from build123d import *

# Parameters (mm, degrees)
SKETCH1_W           = 146.05
SKETCH1_H           = 101.6
BOSS_EXTRUDE1_DEPTH = 2.54
CUT_EXTRUDE1_DEPTH  = 178.931487095
SKETCH4_W           = 40.64
SKETCH4_H           = 95.25
SKETCH4_R           = 4.445
SKETCH4_R_2         = 4.7625
BOSS_EXTRUDE2_DEPTH = 2.54


with BuildPart() as part:
    # Sketch1 → Boss-Extrude1 (new body)
    with BuildSketch(Plane.XY):
        with Locations((73.025, -50.8)):
            Rectangle(SKETCH1_W, SKETCH1_H)
    extrude(amount=BOSS_EXTRUDE1_DEPTH)

    # Sketch2 → Cut-Extrude1 (cut, through all)
    with BuildSketch(Plane.XY):
        with BuildLine():
            Line((80.01, -72.39), (41.91, -72.39))
            Line((41.91, -72.39), (41.91, -80.01))
            Line((41.91, -80.01), (53.34, -99.807340731))
            Line((53.34, -99.807340731), (53.34, -101.6))
            Line((53.34, -101.6), (0, -101.6))
            Line((0, -101.6), (0, -29.21))
            Line((0, -29.21), (-13.136118413, -29.21))
            Line((-13.136118413, -29.21), (-13.136118413, 0))
            Line((-13.136118413, 0), (146.05, 0))
            Line((146.05, 0), (146.05, -5.08))
            Line((146.05, -5.08), (12.065, -5.08))
            ThreePointArc((12.065, -5.08), (0, -17.145), (12.065, -29.21))
            Line((12.065, -29.21), (80.01, -29.21))
            ThreePointArc((80.01, -29.21), (101.6, -50.8), (80.01, -72.39))
        make_face()
        with BuildLine():
            Line((12.065, -12.065), (78.105, -12.065))
            ThreePointArc((78.105, -12.065), (83.185, -17.145), (78.105, -22.225))
            Line((78.105, -22.225), (12.065, -22.225))
            ThreePointArc((12.065, -22.225), (6.985, -17.145), (12.065, -12.065))
        make_face()
        with BuildLine():
            Line((62.23, -79.248), (128.27, -79.248))
            ThreePointArc((128.27, -79.248), (133.35, -84.328), (128.27, -89.408))
            Line((128.27, -89.408), (62.23, -89.408))
            ThreePointArc((62.23, -89.408), (57.15, -84.328), (62.23, -79.248))
        make_face()
    extrude(amount=CUT_EXTRUDE1_DEPTH, mode=Mode.SUBTRACT)

    # Sketch4 → Boss-Extrude2 (add)
    with BuildSketch(Plane.ZY.offset(-146.05)):
        with Locations((22.86, -53.34)):
            Rectangle(SKETCH4_W, SKETCH4_H)
        with Locations((34.29, -29.845)):
            Circle(SKETCH4_R, mode=Mode.SUBTRACT)
        with Locations((13.97, -91.44)):
            Circle(SKETCH4_R_2, mode=Mode.SUBTRACT)
        with BuildLine():
            Line((24.13, -15.748), (24.13, -28.1559))
            ThreePointArc((24.13, -28.1559), (19.177, -33.1089), (14.224, -28.1559))
            Line((14.224, -28.1559), (14.224, -15.748))
            ThreePointArc((14.224, -15.748), (19.177, -10.795), (24.13, -15.748))
        make_face(mode=Mode.SUBTRACT)
        with BuildLine():
            Line((41.91, -78.74), (41.91, -90.17))
            ThreePointArc((41.91, -90.17), (36.195, -95.885), (30.48, -90.17))
            Line((30.48, -90.17), (30.48, -78.74))
            ThreePointArc((30.48, -78.74), (36.195, -73.025), (41.91, -78.74))
        make_face(mode=Mode.SUBTRACT)
    extrude(amount=BOSS_EXTRUDE2_DEPTH)


solid = part.part
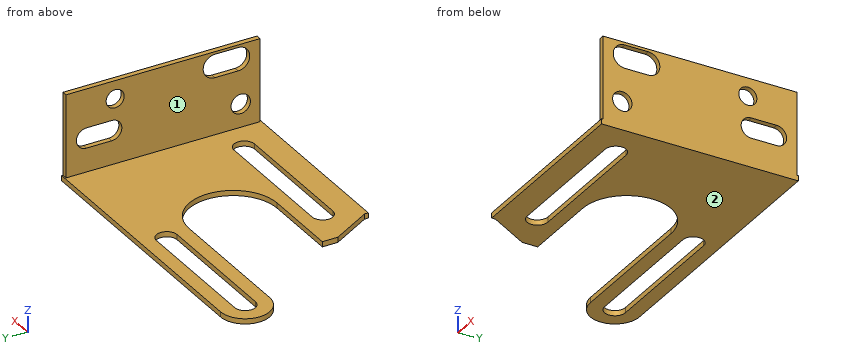
Design review of the part built by this model. Coordinates are the model's own, in mm. Face numbers are marked on the shaded views. A direction names the side the tool comes from. Round coordinates to 2 decimals unless told otherwise and drop trailing zeros. Order: outer loops, then holes, each group sorted by start corner. A loop starts at its lowest first (then second) coordinate and runs counter-clockwise, first axis right, second up.
1) Consider section D-D (y = -50.8). State the section outline as (x, z) points, plus the area to 3 significant figures.
The answers:
outline: (101.6, 0) - (146.05, 0) - (146.05, 43.18) - (143.51, 43.18) - (143.51, 2.54) - (101.6, 2.54) - close
area: 216 mm2
2) Consider section A-A (x = 73.5). State the section outline as (y, z) points (3 decimals).
The answers:
outline: (-101.6, 0) - (-89.408, 0) - (-89.408, 2.54) - (-101.6, 2.54) - close; (-79.248, 0) - (-72.39, 0) - (-72.39, 2.54) - (-79.248, 2.54) - close; (-29.21, 0) - (-22.225, 0) - (-22.225, 2.54) - (-29.21, 2.54) - close; (-12.065, 0) - (-5.08, 0) - (-5.08, 2.54) - (-12.065, 2.54) - close
3) Machinability: for the marked faces 1 and 2, which of the approach directions +Z, -Z, +X, -X, +Y, -Y give a long, thin tool a straight path to every point of the face, cutting with its end or side? Answer none if there is none.
The answers:
face 1: +Z, -X, +Y, -Y
face 2: -Z, +X, -X, +Y, -Y
4) Consider section B-B (y = -77). State the section outline as (x, z) points.
The answers:
outline: (41.91, 0) - (146.05, 0) - (146.05, 30.75) - (143.51, 30.75) - (143.51, 2.54) - (41.91, 2.54) - close; (143.51, 41.64) - (146.05, 41.64) - (146.05, 43.18) - (143.51, 43.18) - close
5) Consider section C-C (x = 108.5). State the section outline as (y, z) points, plus the area to 3 significant figures.
The answers:
outline: (-101.6, 0) - (-89.41, 0) - (-89.41, 2.54) - (-101.6, 2.54) - close; (-79.25, 0) - (-5.08, 0) - (-5.08, 2.54) - (-79.25, 2.54) - close
area: 219 mm2
6) For L1, parallel to Y at x = 145.55, z = 13.97 (1 decimal); L2, parallel to X at y = -39, z = 6; L3, parallel to Z at x = 132, y = -26.5, list the stretches that pass through material, from the lowest coordinate up.
The answers:
L1: y = -101 to -96.2, -86.7 to -5.7
L2: x = 143.51 to 146.05
L3: z = 0 to 2.54
7) Clearance check with flat-ended pins moving along their axes: pin 1 Ø12 at (y, z) = (-76, 14.5) entering from -X; pin 2 Ø2 at (x, z) = (144, 20.5) entering from -Y (3 decimals); pin 3 Ø1.4 at (y, z) = (-101, 1.5) entering from -X. State where each tip first meets the part, or that it passes through.
The answers:
pin 1: stops at x = 143.51
pin 2: stops at y = -100.965
pin 3: stops at x = 53.34
